from build123d import *

# Parameters (mm, degrees)
BOSS_EXTRUDE1_DEPTH = 50
SKETCH5_W           = 30
SKETCH5_H           = 13
CUT_EXTRUDE1_DEPTH  = 135.866600758


with BuildPart() as part:
    # Sketch1 → Boss-Extrude1 (new body)
    with BuildSketch(Plane.XY):
        with BuildLine():
            Line((0, 0), (26, 0))
            Line((26, 0), (26, 12))
            Line((26, 12), (66, 12))
            Line((66, 12), (66, 0))
            Line((66, 0), (92, 0))
            Line((92, 0), (92, 9))
            Line((92, 9), (76, 40))
            Line((76, 40), (71, 40))
            Line((71, 40), (71, 70))
            Line((71, 70), (61, 70))
            ThreePointArc((61, 70), (46, 85), (31, 70))
            Line((31, 70), (21, 70))
            Line((21, 70), (21, 40))
            Line((21, 40), (16, 40))
            Line((16, 40), (0, 9))
            Line((0, 9), (0, 0))
        make_face()
    extrude(amount=BOSS_EXTRUDE1_DEPTH)

    # Sketch5 → Cut-Extrude1 (cut, through all)
    with BuildSketch(Plane(origin=(0, 0, 0), x_dir=(0, 0, -1), z_dir=(1, 0, 0))):
        with Locations((-25, 33.5)):
            Rectangle(SKETCH5_W, SKETCH5_H)
    extrude(amount=CUT_EXTRUDE1_DEPTH, mode=Mode.SUBTRACT)


solid = part.part
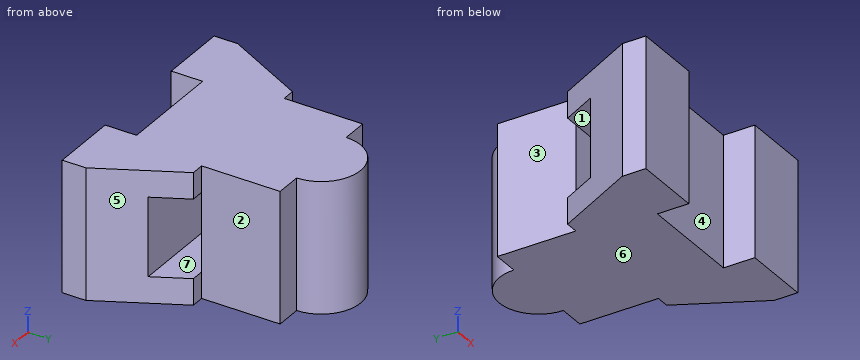
Source: CAD feature listing. Evaluate the final solid. Frame: model axes, mm. Face numbers are marked on the shaded views. A direction names the side the tool comes from. Round coordinates to 2 decimals unless told otherwise and drop trailing zeros. Loops run counter-clockwise (first coordinate to the right, second up) from the corner with the lowest first, then second, coordinate; pieces in that order, holes last. Notation, with made-up numbers: M -10,-28.75 L 45,-28.75 A26 cw 45,-6.75 Z; hole C 62,-4.5 d1. An arc over 180 degrees is marked long. Return JSON: item names as keys, results as strings. Group by question number.
1. Section query B-B on x = 46. Output: boundary loops of the cut face in (y, z), and give its area (3 significant figures).
2. Section query D-D on z = 8.5. Output: boundary loops of the cut face in (x, y).
3. Reachability of the marked faces 1, 2, 3 and 4 from +Z, -Z, +X, -X, +Y, -Y: full face, straight path, thin tool, end or side. Return the list, or none.
4. Section query C-C on y = 34. Output: boundary loops of the cut face in (x, z), and give its area (3 significant figures).
5. Mould query, pull axis Y, two halves, no side actions, for the marked faces 5, 6 and 7. Classes: released by +Y, released by -Y, zero draft, split by the parting line, or undercut.
6. Material intervals for line 1 along X through (y, z) = (4.5, 47.5); line 2 along Y through (x, z) = (62, 16); line 3 along Y through (x, z) = (68, 11.5), sorted ascending. Write a range as from..to.
7. Section query A-A on z = 37. Output: boundary loops of the cut face in (x, y).
8. Pin query (flat end, axial travel): pin 1 (1 mm diameter, centred on x = 28, z = 39, fed in from +Y); pin 2 (6.5 mm diameter, centred on x = 40.5, y = 32.5, fed in from -Z); pin 3 (8 mm diameter, centred on y = 19, z = 21, fed in from -X); pin 4 (2.5 mm diameter, centred on x = 17.5, z = 3, fed in from +Y). Return the tip coordinate at first contact, or that it passes through.
Checks:
{
 "1": {"outline": "M 12,0 L 85,0 L 85,50 L 12,50 Z; hole M 27,10 L 40,10 L 40,40 L 27,40 Z", "area": "3,260 mm²"},
 "2": {"outline": "M 0,0 L 26,0 L 26,12 L 66,12 L 66,0 L 92,0 L 92,9 L 76,40 L 71,40 L 71,70 L 61,70 A15 ccw 31,70 L 21,70 L 21,40 L 16,40 L 0,9 Z"},
 "3": {"face 1": "+X, -X", "face 2": "+Z, -Z, +X, +Y", "face 3": "+Z, -Z, -X, +Y", "face 4": "+Z, -Z, -Y"},
 "4": {"outline": "M 12.9,0 L 79.1,0 L 79.1,10 L 12.9,10 Z; M 12.9,40 L 79.1,40 L 79.1,50 L 12.9,50 Z", "area": "1,320 mm²"},
 "5": {"face 5": "released by +Y", "face 6": "zero draft", "face 7": "undercut"},
 "6": {"line 1": "x = 0..26, 66..92", "line 2": "y = 12..27, 40..70", "line 3": "y = 0..27, 40..70"},
 "7": {"outline": "M 0,0 L 26,0 L 26,12 L 66,12 L 66,0 L 92,0 L 92,9 L 82.71,27 L 9.29,27 L 0,9 Z; M 21,40 L 71,40 L 71,70 L 61,70 A15 ccw 31,70 L 21,70 Z"},
 "8": {"pin 1": "stops at y = 70", "pin 2": "stops at z = 0", "pin 3": "stops at x = 3.1", "pin 4": "stops at y = 40"}
}
